Can you work these out from the model? Positions are in its coordinate system, mm. A direction names the side the tool comes from. Give positions to 0.01 mm unless a question says otherwise; leave off trailing zeros. Write each loop counter-clockwise with the first axis right and the second up, starting at its lowest first coordinate (ties: lowest second). Pieces come first, ordered by that corner, then holes.
```python
from build123d import *

# Parameters (mm, degrees)
SKETCH1_R                = 7.525
SKETCH1_R_2              = 6.025
BOSS_EXTRUDE1_DEPTH      = 2
SKETCH1_5_R              = 22.525
SKETCH1_5_R_2            = 7.525
BOSS_EXTRUDE3_DEPTH      = 3
SKETCH2_R                = 1.75
CUT_EXTRUDE1_DEPTH       = 4.5
CIRPATTERN1_COUNT        = 3
SKETCH9_W                = 60
SKETCH9_H                = 11
BOSS_EXTRUDE7_DEPTH      = 15
BOSS_EXTRUDE7_DEPTH_BACK = 3
CUT_EXTRUDE3_REACH       = 13
SKETCH10_R               = 2.5
FILLET4_R                = 3
FILLET5_R                = 5


with BuildPart() as part:
    # Sketch1 → Boss-Extrude1 (new body)
    with BuildSketch(Plane(origin=(0, 0, 0), x_dir=(1, 0, 0), z_dir=(0, 1, 0))):
        Circle(SKETCH1_R)
        Circle(SKETCH1_R_2, mode=Mode.SUBTRACT)
    extrude(amount=BOSS_EXTRUDE1_DEPTH)

    # Sketch1<5> → Boss-Extrude3 (add)
    with BuildSketch(Plane(origin=(0, 0, 0), x_dir=(1, 0, 0), z_dir=(0, 1, 0))):
        Circle(SKETCH1_5_R)
        Circle(SKETCH1_5_R_2, mode=Mode.SUBTRACT)
    extrude(amount=BOSS_EXTRUDE3_DEPTH)

    # Sketch2 → Cut-Extrude1 (cut)
    with BuildSketch(Plane(origin=(0, 3, 0), x_dir=(1, 0, 0), z_dir=(0, 1, 0))):
        with Locations((0, -15.025)):
            Circle(SKETCH2_R)
    cut_extrude1 = extrude(amount=-CUT_EXTRUDE1_DEPTH, mode=Mode.SUBTRACT)

    # CirPattern1: Cut-Extrude1 ×3 about axis
    cirpattern1_axis = Axis((0, 0, 0), (0, 1, 0))
    for i in range(1, CIRPATTERN1_COUNT):
        add(cut_extrude1.rotate(cirpattern1_axis, i * 360 / CIRPATTERN1_COUNT), mode=Mode.SUBTRACT)

    # Sketch9 → Boss-Extrude7 (add, two sides)
    with BuildSketch(Plane.XZ) as boss_extrude7_sk:
        with Locations((0, -19.5)):
            Rectangle(SKETCH9_W, SKETCH9_H)
    extrude(amount=BOSS_EXTRUDE7_DEPTH)
    extrude(boss_extrude7_sk.sketch, amount=-BOSS_EXTRUDE7_DEPTH_BACK)

    # Sketch10 → Cut-Extrude3 (cut, up to next)
    with BuildSketch(Plane.XY.offset(-14), mode=Mode.PRIVATE) as cut_extrude3_sk1:
        with Locations((-18, -7.5)):
            Circle(SKETCH10_R)
    cut_extrude3_tool1 = extrude(cut_extrude3_sk1.sketch, amount=-CUT_EXTRUDE3_REACH, mode=Mode.PRIVATE) & part.part
    add(cut_extrude3_tool1.solids().sort_by_distance((-18, -7.5, -14))[0], mode=Mode.SUBTRACT)
    # Sketch10 → Cut-Extrude3 (cut, up to next)
    with BuildSketch(Plane.XY.offset(-14), mode=Mode.PRIVATE) as cut_extrude3_sk2:
        with Locations((18, -7.5)):
            Circle(SKETCH10_R)
    cut_extrude3_tool2 = extrude(cut_extrude3_sk2.sketch, amount=-CUT_EXTRUDE3_REACH, mode=Mode.PRIVATE) & part.part
    add(cut_extrude3_tool2.solids().sort_by_distance((18, -7.5, -14))[0], mode=Mode.SUBTRACT)

    # Fillet4
    fillet4_edges = [part.edges().sort_by_distance(p)[0] for p in [
        (-30, -6, -14),
        (30, -6, -14),
    ]]
    fillet(fillet4_edges, radius=FILLET4_R)

    # Fillet5
    fillet5_edges = [part.edges().sort_by_distance(p)[0] for p in [
        (-17.645838745, 1.5, -14),
        (17.645838745, 1.5, -14),
    ]]
    fillet(fillet5_edges, radius=FILLET5_R)


solid = part.part
```
1) For pin 1 Ø4 at (x, z) = (0.5, -4.5) entering from +Y; pin 2 Ø6 at (x, y) = (-12, -11.5) entering from +Z; pin 3 Ø10 at (x, z) = (-16, 0.5) entering from -Y, each with a flat end and sliding along its axis, tell me the tip position at first contact or that it passes through.
Values follow:
pin 1: stops at y = 2
pin 2: stops at z = -14
pin 3: stops at y = 0
2) Suppose I cut it at C-C on z = 0. Write out the boundary of the cut face in (x, y) (3 decimals).
Values follow:
outline: (-22.525, 0) - (-6.025, 0) - (-6.025, 2) - (-7.525, 2) - (-7.525, 3) - (-22.525, 3) - close; (6.025, 0) - (22.525, 0) - (22.525, 3) - (7.525, 3) - (7.525, 2) - (6.025, 2) - close
3) For faces 1 (the face through (-1.631, 2.493, 7.346)), 2 (the face through (15.5, -7.4, -19.4)), which set-ups out of +Z, -Z, +X, -X, +Y, -Y let a thin tool reach every point of the face, with its end or its side?
Values follow:
face 1: +Y
face 2: +Z, -Z
4) Suppose I cut it at D-D on x = 18. Write out the boundary of the cut face in (y, z).
Values follow:
outline: (-15, -25) - (-10, -25) - (-10, -14) - (-15, -14) - close; (-5, -25) - (3, -25) - (3, 13.54) - (0, 13.54) - (0, -14) - (-5, -14) - close
5) If we mould it in two halves opening along Y, with no side actions, what happens to faces 3 (the face through (0, 0, 8)), 4 (the face through (30, -6, -21)), 5 (the face through (-20.5, -7.4, -19.4)), 6 (the face through (-6, 2, -2))? For each: +Y half, -Y half, draft (parallel to the pull), parting line (faces both ways), or undercut.
Values follow:
face 3: -Y half
face 4: draft
face 5: undercut
face 6: +Y half
6) Suppose I cut it at A-A on y = -7.5. Write out the boundary of the cut face in (x, z).
Values follow:
outline: (-30, -25) - (-20.5, -25) - (-20.5, -14) - (-27, -14) arc R3 ccw to (-30, -17) - close; (-15.5, -25) - (15.5, -25) - (15.5, -14) - (-15.5, -14) - close; (20.5, -25) - (30, -25) - (30, -17) arc R3 ccw to (27, -14) - (20.5, -14) - close
7) Suppose I cut it at B-B on x = 0. Write out the boundary of the cut face in (y, z) (3 decimals), plus the area to 3 significant figures.
Values follow:
outline: (-15, -25) - (3, -25) - (3, -7.525) - (2, -7.525) - (2, -6.025) - (0, -6.025) - (0, -14) - (-15, -14) - close; (0, 6.025) - (2, 6.025) - (2, 7.525) - (3, 7.525) - (3, 13.275) - (0, 13.275) - close; (0, 16.775) - (3, 16.775) - (3, 22.525) - (0, 22.525) - close
area: 258 mm2
8) Please list where these lines run through material, in increasing order: L1, parallel to Z at x = 0, y = 2.25 (3 decimals); L2, parallel to Z at x = 0, y = 0.7 (3 decimals); L3, parallel to X at y = -7.25, z = -19.
Values follow:
L1: z = -25 to -7.525, 7.525 to 13.275, 16.775 to 22.525
L2: z = -25 to -6.025, 6.025 to 13.275, 16.775 to 22.525
L3: x = -30 to -20.49, -15.51 to 15.51, 20.49 to 30
